from build123d import *

# Parameters (mm, degrees)
BOSS_EXTRUDE1_DEPTH = 14
FILLET1_R           = 2
SKETCH2_W           = 20
SKETCH2_H           = 5
CUT_EXTRUDE1_DEPTH  = 20


with BuildPart() as part:
    # Sketch1 → Boss-Extrude1 (new body)
    with BuildSketch(Plane(origin=(0, -5, 0), x_dir=(1, 0, 0), z_dir=(0, 1, 0))):
        with BuildLine():
            Line((-111.451663584, 33.777598009), (20.548336416, 33.777598009))
            ThreePointArc((20.548336416, 33.777598009), (24.083870322, 35.242064103), (25.548336416, 38.777598009))
            Line((25.548336416, 38.777598009), (25.548336416, 100.777598009))
            ThreePointArc((25.548336416, 100.777598009), (24.083870322, 104.313131915), (20.548336416, 105.777598009))
            Line((20.548336416, 105.777598009), (-111.451663584, 105.777598009))
            ThreePointArc((-111.451663584, 105.777598009), (-114.98719749, 104.313131915), (-116.451663584, 100.777598009))
            Line((-116.451663584, 100.777598009), (-116.451663584, 38.777598009))
            ThreePointArc((-116.451663584, 38.777598009), (-114.98719749, 35.242064103), (-111.451663584, 33.777598009))
        make_face()
    extrude(amount=BOSS_EXTRUDE1_DEPTH)

    # Fillet1
    fillet1_edges = [part.edges().sort_by_distance(p)[0] for p in [
        (-114.98719749, 9, -35.242064103),
        (-116.451663584, -5, -69.777598009),
        (-114.98719749, -5, -104.313131915),
        (-45.451663584, 9, -33.777598009),
        (24.083870322, 9, -35.242064103),
        (25.548336416, 9, -69.777598009),
        (24.083870322, 9, -104.313131915),
        (-45.451663584, 9, -105.777598009),
        (-114.98719749, 9, -104.313131915),
        (-116.451663584, 9, -69.777598009),
        (-45.451663584, -5, -105.777598009),
        (24.083870322, -5, -104.313131915),
        (25.548336416, -5, -69.777598009),
        (24.083870322, -5, -35.242064103),
        (-45.451663584, -5, -33.777598009),
        (-114.98719749, -5, -35.242064103),
    ]]
    fillet(fillet1_edges, radius=FILLET1_R)

    # Sketch2 → Cut-Extrude1 (cut)
    with BuildSketch(Plane(origin=(25.548336416, 0, 0), x_dir=(0, 0, -1), z_dir=(1, 0, 0))):
        with Locations((87.777598009, 2)):
            Rectangle(SKETCH2_W, SKETCH2_H)
    extrude(amount=-CUT_EXTRUDE1_DEPTH, mode=Mode.SUBTRACT)


solid = part.part
Source: CAD feature listing. Evaluate the final solid. Frame: model axes, mm. A direction names the side the tool comes from. Coordinates: 2 decimals unless noted, no trailing zeros. Order: outer loops, then holes, each group sorted by start corner. A loop starts at its lowest first (then second) coordinate and runs counter-clockwise, first axis right, second up.
Item 1: Pull-direction query (Y, two-part tool) for faces 1 (the face through (16, 2, -97.778)), 2 (the face through (24.04, 1.93, -35.2)), 3 (the face through (-46, 9, -70)); classes: pulls with the +Y half, pulls with the -Y half, needs draft (parallel to the pull), parting line crosses it, or undercut.
Output values:
face 1: undercut
face 2: needs draft
face 3: pulls with the +Y half
Item 2: Cut plane A-A (z = -82.5). Return loops of the section in (x, y).
Output values:
outline: (-116.45, -3) arc R2 ccw to (-114.45, -5) - (23.55, -5) arc R2 ccw to (25.55, -3) - (25.55, -0.5) - (5.55, -0.5) - (5.55, 4.5) - (25.55, 4.5) - (25.55, 7) arc R2 ccw to (23.55, 9) - (-114.45, 9) arc R2 ccw to (-116.45, 7) - close
Item 3: Set-up query: faces 4 (the face through (-45, 2, -105.778)), 5 (the face through (16, 2, -77.778)). Return all of +Z, -Z, +X, -X, +Y, -Y with unobstructed straight access to the full face (end or side cutting, diameter ignored); none if empty.
Output values:
face 4: -Z, +X, -X, +Y, -Y
face 5: +X
Item 4: First-contact query: P1, Ø2.5, axis at y = 2.5, z = -87.5, coming from the +X side. Flat tip, straight axial feed; report the tip coordinate or a pass-through.
Output values:
P1: stops at x = 5.55
Item 5: Material intervals for line 1 (X direction, y = 3.75, z = -81); line 2 (Z direction, x = -50.5, y = -3.5); line 3 (X direction, y = 8, z = -91.5), sorted ascending.
Output values:
line 1: x = -116.45 to 5.55
line 2: z = -105.71 to -33.84
line 3: x = -116.18 to 25.28
